```python
from build123d import *

# Parameters (mm, degrees)
SKETCH1_W           = 279.4
SKETCH1_H           = 415.925
SKETCH1_R           = 9.525
SKETCH1_W_2         = 12.7
SKETCH1_H_2         = 177.8
SKETCH1_W_3         = 114.3
SKETCH1_H_3         = 12.7
BOSS_EXTRUDE3_DEPTH = 3.3528


with BuildPart() as part:
    # Sketch1 → Boss-Extrude3 (new body)
    # profile 1 of 7: a face of its own
    with BuildSketch(Plane.XY):
        Rectangle(SKETCH1_W, SKETCH1_H)
        with Locations((117.475, -122.2375)):
            Circle(SKETCH1_R, mode=Mode.SUBTRACT)
        with Locations((117.475, 122.2375)):
            Circle(SKETCH1_R, mode=Mode.SUBTRACT)
        with Locations((-117.475, -122.2375)):
            Circle(SKETCH1_R, mode=Mode.SUBTRACT)
        with Locations((-117.475, 122.2375)):
            Circle(SKETCH1_R, mode=Mode.SUBTRACT)
    # profile 2 of 7: a face of its own
    with BuildSketch(Plane.XY):
        with Locations((-146.05, 103.98125)):
            Rectangle(SKETCH1_W_2, SKETCH1_H_2)
    # profile 3 of 7: a face of its own
    with BuildSketch(Plane.XY):
        with Locations((-73.025, 214.3125)):
            Rectangle(SKETCH1_W_3, SKETCH1_H_3)
    # profile 4 of 7: a face of its own
    with BuildSketch(Plane.XY):
        with Locations((-146.05, -103.98125)):
            Rectangle(SKETCH1_W_2, SKETCH1_H_2)
    # profile 5 of 7: a face of its own
    with BuildSketch(Plane.XY):
        with Locations((73.025, 214.3125)):
            Rectangle(SKETCH1_W_3, SKETCH1_H_3)
    # profile 6 of 7: a face of its own
    with BuildSketch(Plane.XY):
        with Locations((-73.025, -214.3125)):
            Rectangle(SKETCH1_W_3, SKETCH1_H_3)
    # profile 7 of 7: a face of its own
    with BuildSketch(Plane.XY):
        with Locations((73.025, -214.3125)):
            Rectangle(SKETCH1_W_3, SKETCH1_H_3)
    extrude(amount=BOSS_EXTRUDE3_DEPTH)


solid = part.part
```
Geometry: final body of the model. Coordinates: model frame, mm. Coordinates: 2 decimals unless noted, no trailing zeros. Order: outer loops, then holes, each group sorted by start corner. A loop starts at its lowest first (then second) coordinate and runs counter-clockwise, first axis right, second up. Notation, with made-up numbers: (40, 22) - (91, 22) arc R16 ccw to (91, 35) - close; hole circle Ø6 at (-2, 76.25). An arc over 180 degrees is marked (long way). Write each question's results on one line, items separated by ' | '.
1) Section B-B, the plane z = 0.95. State how many separate pieces and enclosed holes the cut face has, plus the area to 3 significant figures.
Results list:
separate pieces: 1 | enclosed holes: 4 | area: 125,000 mm^2
2) Section C-C, the plane x = 114.5. Return loops of the section in (y, z).
Results list:
outline: (-220.66, 0) - (-131.29, 0) - (-131.29, 3.35) - (-220.66, 3.35) - close; (-113.19, 0) - (113.19, 0) - (113.19, 3.35) - (-113.19, 3.35) - close; (131.29, 0) - (220.66, 0) - (220.66, 3.35) - (131.29, 3.35) - close
3) Section D-D, the plane x = 1.5. Return loops of the section in (y, z).
Results list:
outline: (-207.96, 0) - (207.96, 0) - (207.96, 3.35) - (-207.96, 3.35) - close
4) Line query: line 1 (Y direction, x = 112, z = 0.7); line 2 (Y direction, x = -139.5, z = 2.3). Output: solid intervals per line, ascending. Write a range as from..to.
Results list:
line 1: -220.66..-130.03, -114.44..114.44, 130.03..220.66 | line 2: -207.96..207.96
5) Pin query (flat end, axial travel): pin 1 (1.7 mm diameter, centred on y = -217, z = 1, fed in from -X) (3 decimals); pin 2 (1 mm diameter, centred on x = -4.5, z = 1, fed in from -Y); pin 3 (1.7 mm diameter, centred on x = 2, z = 1, fed in from +Y). Return the tip coordinate at first contact, or that it passes through.
Results list:
pin 1: x = -130.175 | pin 2: y = -207.96 | pin 3: y = 207.96
6) Pull-direction query (Y, two-part tool) for faces 1 (the flat face through (-8, 3, 3.353)), 2 (the cylindrical face through (109.916, -128.033, 1.653)); classes: pulls with the +Y half, pulls with the -Y half, needs draft (parallel to the pull), parting line crosses it, or undercut.
Results list:
face 1: needs draft | face 2: undercut
7) Section A-A, the plane x = -113. Return loops of the section in (y, z).
Results list:
outline: (-220.66, 0) - (-130.65, 0) - (-130.65, 3.35) - (-220.66, 3.35) - close; (-113.83, 0) - (113.83, 0) - (113.83, 3.35) - (-113.83, 3.35) - close; (130.65, 0) - (220.66, 0) - (220.66, 3.35) - (130.65, 3.35) - close
